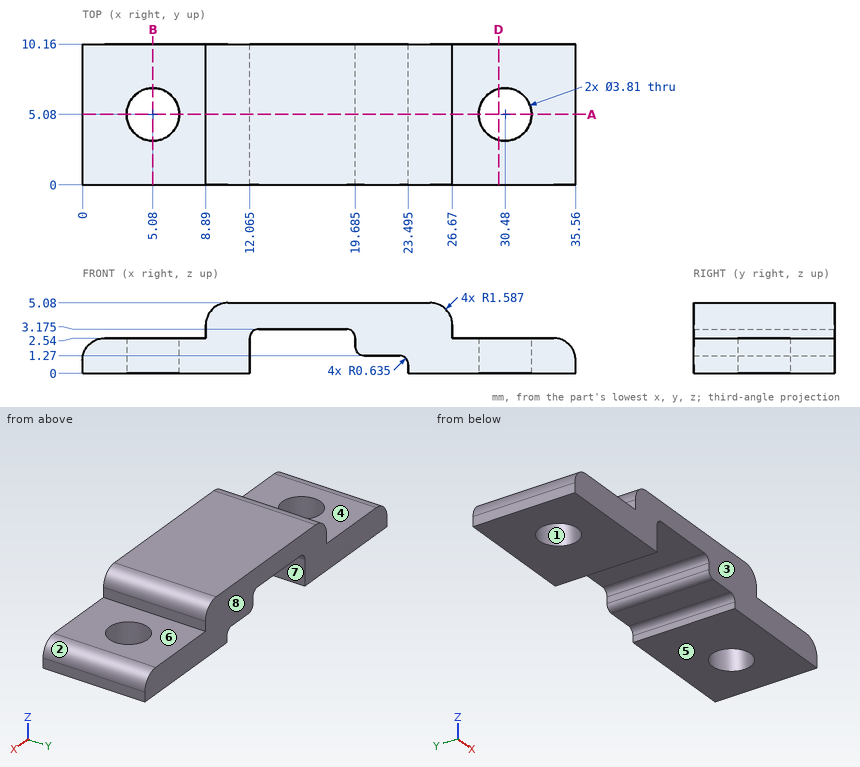
The figure shows three views and two pictorial views of one solid part (mm, origin at its lowest corner). Answer the questions. A direction names the side the tool comes from. Round coordinates to 2 decimals unless told otherwise and drop trailing zeros. Order: outer loops, then holes, each group sorted by start corner. A loop starts at its lowest first (then second) coordinate and runs counter-clockwise, first axis right, second up. Notation, with made-up numbers: (-25, 77) - (-13, 77) arc R21 ccw to (-13, 103) - close; hole circle Ø6 at (-19, -7.75). An arc over 180 degrees is marked (long way). Write item = value, one per line. Start each with the question number.
1) Section B-B, the plane x = 5.08 is taken. Write down the section's boundary in (y, z) (1 decimal).
2) Section A-A, the plane y = 5.08 is taken. Count the separate pieces of the cut face and the enclosed holes in it.
3) Straight lines are drawn through the part: L1, parallel to Y at x = 30.48, z = 0.55 (1 decimal); L2, parallel to X at y = 3.5, z = 1.5 (1 decimal); L3, parallel to X at y = 5.08, z = 0.8 (1 decimal). For each, find the intervals that lie inside material, in ascending order.
4) For a pull along Y with two mould halves and no side action, classify the marked faces 1, 2 and 3 as released by +Y, released by -Y, zero draft, split by the parting line, or undercut.
5) For the marked faces 4, 5, 6, 7 and 8, determine the directions among +Z, -Z, +X, -X, +Y, -Y from which every point of the face is accessible in a straight line to the end or side of a thin tool.
6) Section D-D, the plane x = 30 is taken. Write down the section's boundary in (y, z).
7) Given pin 1 (3.5 mm diameter, centred on x = 5.08, y = 5.08, fed in from +Z); pin 2 (1.5 mm diameter, centred on y = 8.5, z = 3, fed in from -X) (1 decimal); pin 3 (1.9 mm diameter, centred on x = 16, y = 3, fed in from -Z) (1 decimal); pin 4 (3.5 mm diameter, centred on x = 5.5, y = 3, fed in from +Z), each flat-ended and moving along its own axis, determine where each tip first touches the part or whether it passes through.
Results list:
q1.outline = (0, 0) - (3.2, 0) - (3.2, 2.5) - (0, 2.5) - close; (7, 0) - (10.2, 0) - (10.2, 2.5) - (7, 2.5) - close
q2.separate_pieces = 3
q2.enclosed_holes = 0
q3.L1 = 0 to 3.2, 7 to 10.2
q3.L2 = 0.1 to 4, 6.1 to 12.1, 19.8 to 29.4, 31.5 to 35.5
q3.L3 = 0 to 3.2, 7 to 12.1, 23.5 to 28.6, 32.4 to 35.6
q4.face_1 = undercut
q4.face_2 = zero draft
q4.face_3 = released by -Y
q5.face_4 = +Z, -X, +Y, -Y
q5.face_5 = -Z, +X, -X, +Y, -Y
q5.face_6 = +Z, +X, +Y, -Y
q5.face_7 = -Z, +Y, -Y
q5.face_8 = +Z, -Z, +X, -X, +Y
q6.outline = (0, 0) - (3.24, 0) - (3.24, 2.54) - (0, 2.54) - close; (6.92, 0) - (10.16, 0) - (10.16, 2.54) - (6.92, 2.54) - close
q7.pin_1 = through
q7.pin_2 = 0.7
q7.pin_3 = 3.2
q7.pin_4 = 2.54
